```python
from build123d import *

# Parameters (mm, degrees)
F0_W      = 101.6
F0_H      = 76.2
F1_DEPTH  = 2.54
F2_W      = 101.6
F2_H      = 50.8
F3_DEPTH  = 21.59
F4_R      = 5.08
F5_W      = 96.52
F5_H      = 19.05
F6_DEPTH  = 48.26
F7_R      = 5.08
F8_R      = 5.08
F9_R      = 5.08
F11_W     = 81.28
F11_H     = 25.4
F12_DEPTH = 21.59
F13_R     = 2.413
F14_DEPTH = 2.541


# Not quite as in the source:
# - a feature of the source that left no trace in its solid (it failed there, or was rolled back) is left out


with BuildPart() as f1:
    # F0 (on Front) → F1 (new body)
    with BuildSketch(Plane.XZ):
        with Locations((50.8, 38.1)):
            Rectangle(F0_W, F0_H)
    extrude(amount=F1_DEPTH)

    # F2 (on face) → F3 (join)
    with BuildSketch(Plane.XZ.offset(2.54)):
        with Locations((50.8, 25.4)):
            Rectangle(F2_W, F2_H)
    extrude(amount=F3_DEPTH)

    # F4
    f4_edges = [f1.edges().sort_by_distance(p)[0] for p in [
        (101.6, -1.27, 76.2),
        (101.6, -12.065, 0),
        (0, -12.065, 0),
        (0, -1.27, 76.2),
    ]]
    fillet(f4_edges, radius=F4_R)

    # F5 (on face) → F6 (cut)
    with BuildSketch(Plane.XY.offset(50.8)):
        with Locations((50.8, -12.065)):
            Rectangle(F5_W, F5_H)
    extrude(amount=-F6_DEPTH, mode=Mode.SUBTRACT)

    # F7
    f7_edges = [f1.edges().sort_by_distance(p)[0] for p in [
        (101.6, -24.13, 27.94),
    ]]
    fillet(f7_edges, radius=F7_R)

    # F8
    f8_edges = [f1.edges().sort_by_distance(p)[0] for p in [
        (99.06, -21.59, 26.67),
    ]]
    fillet(f8_edges, radius=F8_R)

    # F9
    f9_edges = [f1.edges().sort_by_distance(p)[0] for p in [
        (2.54, -21.59, 26.67),
    ]]
    fillet(f9_edges, radius=F9_R)

    # F11 (on face) → F12 (cut, through all)
    with BuildSketch(Plane.XZ.offset(24.13)):
        with Locations((50.8, 21.59)):
            Rectangle(F11_W, F11_H)
    extrude(amount=-F12_DEPTH, mode=Mode.SUBTRACT)

    # F13 (on face) → F14 (cut, through all)
    with BuildSketch(Plane.XZ.offset(2.54)):
        with Locations((91.44, 66.04)):
            Circle(F13_R)
        with Locations((10.16, 66.04)):
            Circle(F13_R)
    extrude(amount=-F14_DEPTH, mode=Mode.SUBTRACT)


solid = f1.part
```
Check sheet for the modelled part. Datum: model origin and axes. Units: mm. A direction names the side the tool comes from. Round coordinates to 2 decimals unless told otherwise and drop trailing zeros. Order: outer loops, then holes, each group sorted by start corner. A loop starts at its lowest first (then second) coordinate and runs counter-clockwise, first axis right, second up.
1) Section check C-C (z = 43). Record the boundary of the cut face in (x, y), and give its area (3 significant figures).
2) Mould release check, pull along Y, two halves, no side actions. Record for faces 4 (the cylindrical face through (4.068, -20.141, 26.332)), 5 (the cylindrical face through (93.742, -1.288, 66.765)), 6 (the flat face through (50, -2.54, 40)), 7 (the flat face through (50, 0, 39)): +Y half, -Y half, draft (parallel to the pull), parting line (faces both ways), or undercut.
3) Section check D-D (y = -9.25). Record the boundary of the cut face in (x, z).
4) Section check A-A (x = 80.5). Record the boundary of the cut face in (y, z), and give its area (3 significant figures).
5) Section check B-B (z = 66.04). Record the boundary of the cut face in (x, y).
6) Tool access check on faces 1 (the flat face through (50, -12, 2.54)), 2 (the cylindrical face through (100.072, -22.681, 28.26)), 3 (the flat face through (50, -23, 34.29)). Record the directions out of +Z, -Z, +X, -X, +Y, -Y that give a thin tool (end or side, any length) a straight path to the whole face; none if there is none.
7) Scan lines: line 1 (Y direction, x = 80, z = 39.5); line 2 (Z direction, x = 91.44, y = -1.95); line 3 (X direction, y = -14.5, z = 7). Record each from-to range of solid material in increasing order.
8) Go/stop test with flat-tipped pins: pin 1 Ø3 at (x, y) = (54.5, -23.5) entering from -Z; pin 2 Ø12 at (y, z) = (-21.5, 57.5) entering from +X; pin 3 Ø4 at (x, y) = (66, -21.5) entering from +Z; pin 4 Ø8 at (x, y) = (21.5, -13.5) entering from +Z. Record where each tip stops, or that it passes through.
Result:
1. outline: (0, -19.05) arc R5.08 ccw to (5.08, -24.13) - (96.52, -24.13) arc R5.08 ccw to (101.6, -19.05) - (101.6, 0) - (0, 0) - close; hole (2.54, -16.51) arc R5.08 ccw to (7.62, -21.59) - (93.98, -21.59) arc R5.08 ccw to (99.06, -16.51) - (99.06, -2.54) - (2.54, -2.54) - close
1. area: 613 mm2
2. face 4: undercut
2. face 5: draft
2. face 6: undercut
2. face 7: +Y half
3. outline: (0, 5.08) arc R5.08 ccw to (5.08, 0) - (96.52, 0) arc R5.08 ccw to (101.6, 5.08) - (101.6, 50.8) - (99.06, 50.8) - (99.06, 2.54) - (2.54, 2.54) - (2.54, 50.8) - (0, 50.8) - close
4. outline: (-24.13, 5.08) arc R5.08 ccw to (-19.05, 0) - (0, 0) - (0, 76.2) - (-2.54, 76.2) - (-2.54, 2.54) - (-21.59, 2.54) - (-21.59, 8.89) - (-24.13, 8.89) - close; (-24.13, 34.29) - (-21.59, 34.29) - (-21.59, 50.8) - (-24.13, 50.8) - close
4. area: 301 mm2
5. outline: (0, -2.54) - (7.75, -2.54) - (7.75, 0) - (0, 0) - close; (12.57, -2.54) - (89.03, -2.54) - (89.03, 0) - (12.57, 0) - close; (93.85, -2.54) - (101.6, -2.54) - (101.6, 0) - (93.85, 0) - close
6. face 1: +Z
6. face 2: +Z, -Z, +X, -Y
6. face 3: -Y
7. line 1: y = -24.13 to -21.59, -2.54 to 0
7. line 2: z = 0 to 63.63, 68.45 to 76.2
7. line 3: x = 0 to 2.54, 99.06 to 101.6
8. pin 1: stops at z = 0.94
8. pin 2: passes through
8. pin 3: stops at z = 50.8
8. pin 4: stops at z = 2.54
